Model file for the job. Use its own axes, mm. A direction names the side the tool comes from. Round coordinates to 2 decimals unless told otherwise and drop trailing zeros. Loops run counter-clockwise (first coordinate to the right, second up) from the corner with the lowest first, then second, coordinate; pieces in that order, holes last. Notation, with made-up numbers: (-2, 50) - (53, 50) arc R26 ccw to (53, 80) - close; hole circle Ø1 at (73, 8.5). An arc over 180 degrees is marked (long way). Answer as a JSON object with one key per item and string values.
from build123d import *

# Parameters (mm, degrees)
EXTRUDE_2_DEPTH     = 15
CUT_EXTRUDE_2_DEPTH = 13
SKETCH_5_R          = 6.5
CUT_EXTRUDE_3_DEPTH = 0.5
SKETCH_6_R          = 6.5
CUT_EXTRUDE_5_DEPTH = 0.5
SKETCH_7_R          = 6.5
CUT_EXTRUDE_8_DEPTH = 0.5


with BuildPart() as part:
    # 草图1 → 凸台-拉伸2 (new body)
    with BuildSketch(Plane.XY):
        Polygon((0, 24.697120967), (-28.517778878, -24.697120967), (28.517778878, -24.697120967), align=None)
    extrude(amount=EXTRUDE_2_DEPTH)

    # 草图4 → 切除-拉伸2 (cut)
    with BuildSketch(Plane.XY):
        with BuildLine():
            Line((-13.473817403, -3.562999264), (-13.473817403, -20.062999264))
            ThreePointArc((-13.473817403, -20.062999264), (-12.456359842, -22.519359106), (-10, -23.536816667))
            Line((-10, -23.536816667), (10, -23.536816667))
            ThreePointArc((10, -23.536816667), (12.456359842, -22.519359106), (13.473817403, -20.062999264))
            Line((13.473817403, -20.062999264), (13.473817403, -3.562999264))
            ThreePointArc((13.473817403, -3.562999264), (10.667568819, 4.667840965), (3.417761445, 9.470137814))
            Line((3.417761445, 9.470137814), (2.376312346, 9.700444286))
            ThreePointArc((2.376312346, 9.700444286), (0, 10.502453106), (-2.376312346, 9.700444286))
            Line((-2.376312346, 9.700444286), (-3.417761445, 9.470137814))
            ThreePointArc((-3.417761445, 9.470137814), (-10.667568819, 4.667840965), (-13.473817403, -3.562999264))
        make_face()
    extrude(amount=CUT_EXTRUDE_2_DEPTH, mode=Mode.SUBTRACT)

    # 草图5 → 切除-拉伸3 (cut)
    with BuildSketch(Plane.XZ.offset(24.697120967)):
        with Locations((0, 7.5)):
            Circle(SKETCH_5_R)
    extrude(amount=-CUT_EXTRUDE_3_DEPTH, mode=Mode.SUBTRACT)

    # 草图6 → 切除-拉伸5 (cut)
    with BuildSketch(Plane(origin=(-14.258889439, 0, 0), x_dir=(0.5, 0.866025404, 0), z_dir=(0.866025404, -0.5, 0))):
        with Locations((0, 7.5)):
            Circle(SKETCH_6_R)
    extrude(amount=CUT_EXTRUDE_5_DEPTH, mode=Mode.SUBTRACT)

    # 草图7 → 切除-拉伸8 (cut)
    with BuildSketch(Plane(origin=(14.258889439, 0, 0), x_dir=(0.5, -0.866025404, 0), z_dir=(-0.866025404, -0.5, 0))):
        with Locations((0, 7.5)):
            Circle(SKETCH_7_R)
    extrude(amount=CUT_EXTRUDE_8_DEPTH, mode=Mode.SUBTRACT)


solid = part.part
1) Slice it at A-A on z = 11.75. List the corners of the cut face in (x, y), then the cut area to 3 significant figures.
Values follow:
{"outline": "(-28.52, -24.7) - (-4.92, -24.7) - (-4.92, -24.2) - (4.92, -24.2) - (4.92, -24.7) - (28.52, -24.7) - (16.72, -4.26) - (16.28, -4.51) - (11.37, 4.01) - (11.8, 4.26) - (0, 24.7) - (-11.8, 4.26) - (-11.37, 4.01) - (-16.28, -4.51) - (-16.72, -4.26) - close; hole (-13.47, -20.06) arc R3.47 ccw to (-10, -23.54) - (10, -23.54) arc R3.47 ccw to (13.47, -20.06) - (13.47, -3.56) arc R13.47 ccw to (3.42, 9.47) - (2.38, 9.7) arc R3.92 ccw to (-2.38, 9.7) - (-3.42, 9.47) arc R13.47 ccw to (-13.47, -3.56) - close", "area": "574 mm²"}
2) Slice it at B-B on y = -9.5. List the corners of the cut face in (x, z).
Values follow:
{"outline": "(-19.74, 0) - (-13.47, 0) - (-13.47, 13) - (13.47, 13) - (13.47, 0) - (19.74, 0) - (19.74, 15) - (-19.74, 15) - close"}
3) Two-plate mould, pull along Y, no slides. Class faces 1 (the flat face through (0, -24.197, 8)), 2 (the cylindrical face through (10.74, 4.57, 6.41)), 3 (the flat face through (0, -5, 15)): pulls with the +Y half, pulls with the -Y half, needs draft (parallel to the pull), parting line crosses it, or undercut.
Values follow:
{"face 1": "pulls with the -Y half", "face 2": "undercut", "face 3": "needs draft"}
4) Probe probe 1 along Z at (x, y) = (0, -24.3); probe 2 along Y at (x, z) = (3.5, 3); probe 3 along X at (y, z) = (-17.5, 10.5). List the from-to ranges inside material, lowest first.
Values follow:
{"probe 1": "0 to 1, 14 to 15", "probe 2": "-24.2 to -23.54, 9.45 to 18.63", "probe 3": "-24.36 to -13.47, 13.47 to 24.36"}
5) Drop flat-ended pins along their axis: P1, Ø6.5, axis at y = -9, z = 6.5, coming from the +X side; P2, Ø2, axis at y = -15.5, z = 7, coming from the -X side; P3, Ø3, axis at y = -16.5, z = 6.5, coming from the +X side. Give the stop position or say it passes through.
Values follow:
{"P1": "x = 21.33", "P2": "x = -23.79", "P3": "x = 24.65"}
6) Slice it at D-D on z = 7.5. List the corners of the cut face in (x, y), then the cut area to 3 significant figures.
Values follow:
{"outline": "(-28.52, -24.7) - (-6.5, -24.7) - (-6.5, -24.2) - (6.5, -24.2) - (6.5, -24.7) - (28.52, -24.7) - (17.51, -5.63) - (17.08, -5.88) - (10.58, 5.38) - (11.01, 5.63) - (0, 24.7) - (-11.01, 5.63) - (-10.58, 5.38) - (-17.08, -5.88) - (-17.51, -5.63) - close; hole (-13.47, -20.06) arc R3.47 ccw to (-10, -23.54) - (10, -23.54) arc R3.47 ccw to (13.47, -20.06) - (13.47, -3.56) arc R13.47 ccw to (3.42, 9.47) - (2.38, 9.7) arc R3.92 ccw to (-2.38, 9.7) - (-3.42, 9.47) arc R13.47 ccw to (-13.47, -3.56) - close", "area": "569 mm²"}
7) Tool access for faces 4 (the flat face through (-10.891, 5.834, 7.395)), 5 (the cylindrical face through (-4.791, -24.451, 11.893)), 6 (the cylindrical face through (-10.59, 4.77, 6.41)): list every direction of +Z, -Z, +X, -X, +Y, -Y with a clear straight run to the whole face (end or side of a thin tool).
Values follow:
{"face 4": "+Z, -Z, -X, +Y", "face 5": "-Y", "face 6": "-Z"}
8) Slice it at C-C on x = -1. List the corners of the cut face in (y, z), then the cut area to 3 significant figures.
Values follow:
{"outline": "(-24.7, 0) - (-23.54, 0) - (-23.54, 13) - (10.37, 13) - (10.37, 0) - (22.97, 0) - (22.97, 15) - (-24.7, 15) - (-24.7, 13.92) - (-24.2, 13.92) - (-24.2, 1.08) - (-24.7, 1.08) - close", "area": "268 mm²"}
